from build123d import *

# Parameters (mm, degrees)
F1_DEPTH = 5


with BuildPart() as f1:
    # F0 (on Top) → F1 (new body)
    with BuildSketch(Plane.XY):
        with BuildLine():
            ThreePointArc((3.434505, 1.711893), (0, -3.8375), (-3.434505, 1.711893))
            ThreePointArc((-3.434505, 1.711893), (-3.418863, 1.89548), (-3.533252, 2.039924))
            Line((-3.533252, 2.039924), (-5.055423, 2.91875))
            ThreePointArc((-5.055423, 2.91875), (-5.638592, 1.510856), (-5.8375, 0))
            ThreePointArc((-5.8375, 0), (-4.127736, -4.127736), (0, -5.8375))
            ThreePointArc((0, -5.8375), (4.127736, -4.127736), (5.8375, 0))
            ThreePointArc((5.8375, 0), (5.638592, 1.510856), (5.055423, 2.91875))
            Line((5.055423, 2.91875), (3.533252, 2.039924))
            ThreePointArc((3.533252, 2.039924), (3.418863, 1.89548), (3.434505, 1.711893))
        make_face()
        with BuildLine():
            ThreePointArc((0, -5.8375), (-4.127736, -4.127736), (-5.8375, 0))
            Line((-5.8375, 0), (-5.8375, -3.8375))
            ThreePointArc((-5.8375, -3.8375), (-5.251714, -5.251714), (-3.8375, -5.8375))
            Line((-3.8375, -5.8375), (0, -5.8375))
        make_face()
        with BuildLine():
            Line((5.8375, -3.8375), (5.8375, 0))
            ThreePointArc((5.8375, 0), (4.127736, -4.127736), (0, -5.8375))
            Line((0, -5.8375), (3.8375, -5.8375))
            ThreePointArc((3.8375, -5.8375), (5.251714, -5.251714), (5.8375, -3.8375))
        make_face()
    extrude(amount=F1_DEPTH)


solid = f1.part
Could you check a few things on this model? Use its own coordinates, in mm. A direction names the side the tool comes from. Coordinates: 2 decimals unless noted, no trailing zeros. Loops run counter-clockwise (first coordinate to the right, second up) from the corner with the lowest first, then second, coordinate; pieces in that order, holes last.
1. I need wall thicknesses on L1, parallel to X at y = 0, z = 2.8; L2, parallel to X at y = -1.25, z = 3.8; L3, parallel to Y at x = 4.5, z = 2.3. Which ranges of each line are inside material? Lowest first, please.
2. Imagine slicing it at A-A (y = -2.75). Please give me the cut outline in (x, z).
3. We'd pull the mould along X, two halves only. Please class faces 1 (the face through (5.2, -5.3, 2.5)), 2 (the face through (-5.838, -2, 2)), 3 (the face through (0.109, -3.836, 2.465)): released by +X, released by -X, zero draft, split by the parting line, or undercut.
4. For faces 4 (the face through (-4.28, 2.47, 2.46)), 5 (the face through (0, -4, 5)), which set-ups out of +Z, -Z, +X, -X, +Y, -Y let a thin tool reach every point of the face, with its end or its side?
5. Imagine slicing it at D-D (y = -0.75). Please give me the cut outline in (x, z).
6. Imagine slicing it at B-B (x = 0). Please give me the cut outline in (y, z).
Computed values:
1. L1: x = -5.84 to -3.84, 3.84 to 5.84
1. L2: x = -5.84 to -3.63, 3.63 to 5.84
1. L3: y = -5.72 to 2.6
2. outline: (-5.84, 0) - (-2.68, 0) - (-2.68, 5) - (-5.84, 5) - close; (2.68, 0) - (5.84, 0) - (5.84, 5) - (2.68, 5) - close
3. face 1: released by +X
3. face 2: released by -X
3. face 3: undercut
4. face 4: +Z, -Z, +Y
4. face 5: +Z, +X, -X, +Y, -Y
5. outline: (-5.84, 0) - (-3.76, 0) - (-3.76, 5) - (-5.84, 5) - close; (3.76, 0) - (5.84, 0) - (5.84, 5) - (3.76, 5) - close
6. outline: (-5.84, 0) - (-3.84, 0) - (-3.84, 5) - (-5.84, 5) - close
